```python
from build123d import *

# Parameters (mm, degrees)
F0_W      = 580
F0_H      = 322
F1_DEPTH  = 17.5
F2_W      = 85
F2_H      = 140
F3_DEPTH  = 25
F4_W      = 322
F4_H      = 35
F5_DEPTH  = 30
F6_W      = 20
F6_H      = 302
F7_DEPTH  = 35.001
F8_W      = 322
F8_H      = 35
F9_DEPTH  = 40
F10_W     = 30
F10_H     = 302
F11_DEPTH = 35.001
F13_W     = 630
F13_H     = 302
F14_DEPTH = 5


with BuildPart() as f1:
    # F0 (on Top) → F1 (new body, symmetric)
    with BuildSketch(Plane.XY):
        Rectangle(F0_W, F0_H)
    extrude(amount=F1_DEPTH, both=True)

    # F2 (on Top) → F3 (cut, symmetric)
    with BuildSketch(Plane.XY):
        with Locations((237.5, -81)):
            Rectangle(F2_W, F2_H)
        with Locations((142.5, -81)):
            Rectangle(F2_W, F2_H)
        with Locations((47.5, -81)):
            Rectangle(F2_W, F2_H)
        with Locations((-47.5, -81)):
            Rectangle(F2_W, F2_H)
        with Locations((-142.5, -81)):
            Rectangle(F2_W, F2_H)
        with Locations((142.5, 81)):
            Rectangle(F2_W, F2_H)
        with Locations((237.5, 81)):
            Rectangle(F2_W, F2_H)
        with Locations((47.5, 81)):
            Rectangle(F2_W, F2_H)
        with Locations((-142.5, 81)):
            Rectangle(F2_W, F2_H)
        with Locations((-47.5, 81)):
            Rectangle(F2_W, F2_H)
        with Locations((-237.5, 81)):
            Rectangle(F2_W, F2_H)
        with Locations((-237.5, -81)):
            Rectangle(F2_W, F2_H)
    extrude(amount=F3_DEPTH, both=True, mode=Mode.SUBTRACT)


with BuildPart() as f5:
    # F4 (on face) → F5 (new body)
    with BuildSketch(Plane(origin=(-290, 0, 0), x_dir=(0, -1, 0), z_dir=(-1, 0, 0))):
        Rectangle(F4_W, F4_H)
    extrude(amount=F5_DEPTH)

    # F6 (on face) → F7 (cut, through all)
    with BuildSketch(Plane(origin=(0, 0, -17.5), x_dir=(1, 0, 0), z_dir=(0, 0, -1))):
        with Locations((-300, 0)):
            Rectangle(F6_W, F6_H)
    extrude(amount=-F7_DEPTH, mode=Mode.SUBTRACT)


with BuildPart() as f9:
    # F8 (on face) → F9 (new body)
    with BuildSketch(Plane.YZ.offset(290)):
        Rectangle(F8_W, F8_H)
    extrude(amount=F9_DEPTH)

    # F10 (on face) → F11 (cut, through all)
    with BuildSketch(Plane(origin=(0, 0, -17.5), x_dir=(1, 0, 0), z_dir=(0, 0, -1))):
        with Locations((305, 0)):
            Rectangle(F10_W, F10_H)
    extrude(amount=-F11_DEPTH, mode=Mode.SUBTRACT)


with BuildPart() as f5_1:
    add(f5.part)

    # F12: union F1, F9
    add(f1.part)
    add(f9.part)

    # F13 (on face) → F14 (join)
    with BuildSketch(Plane(origin=(0, 0, -17.5), x_dir=(1, 0, 0), z_dir=(0, 0, -1))):
        with Locations((5, 0)):
            Rectangle(F13_W, F13_H)
    extrude(amount=-F14_DEPTH)


solid = f5_1.part
```
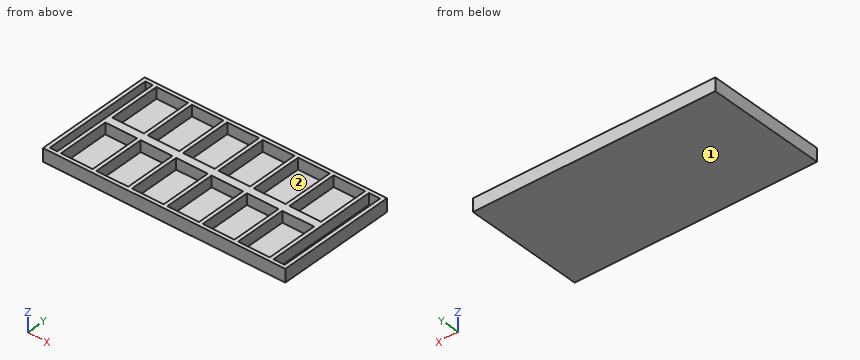
Geometry check sheet. Reference: the model listing, model coordinates, mm. Face numbers are marked on the shaded views. Coordinates: 2 decimals unless noted, no trailing zeros. Order: outer loops, then holes, each group sorted by start corner. A loop starts at its lowest first (then second) coordinate and runs counter-clockwise, first axis right, second up. Notation, with made-up numbers: (21.5, -31) - (79.5, -31) arc R34 cw to (79.5, 5) - close; hole circle Ø7 at (-13, 7.5). An arc over 180 degrees is marked (long way). Answer as a JSON object with one key per item and string values. Group by question number.
Item 1: Depth check by flat-ended pin: pin 1 Ø12 at (x, y) = (-109.5, 82.5) entering from +Z. Enter the tip coordinate at first touch or a pass-through.
Item 2: Scan lines: probe 1 along Y at (x, z) = (210.5, 14); probe 2 along Y at (x, z) = (292, -3); probe 3 along Z at (x, y) = (67, 34). Record each from-to range of solid material in increasing order.
Item 3: Sectioned sample at A-A, the plane x = 113.5. Record the cut outline in (y, z), and give its area (3 significant figures).
Item 4: Draft check along X on the marked faces 1 and 2. Enter one of: +X half, -X half, draft (parallel to the pull), parting line (faces both ways), or undercut.
Item 5: Sectioned sample at B-B, the plane z = 2.5. Give the number of separate pieces and of enclosed holes in the cut face, and give its area (3 significant figures).
Resolved:
{
 "1": {"pin 1": "z = -12.5"},
 "2": {"probe 1": "-161 to -151, -11 to 11, 151 to 161", "probe 2": "-161 to -151, 151 to 161", "probe 3": "-17.5 to -12.5"},
 "3": {"outline": "(-161, -17.5) - (161, -17.5) - (161, 17.5) - (151, 17.5) - (151, -12.5) - (11, -12.5) - (11, 17.5) - (-11, 17.5) - (-11, -12.5) - (-151, -12.5) - (-151, 17.5) - (-161, 17.5) - close", "area": "2,870 mm^2"},
 "4": {"face 1": "draft", "face 2": "undercut"},
 "5": {"separate pieces": "1", "enclosed holes": "14", "area": "51,400 mm^2"}
}
